from build123d import *

# Parameters (mm, degrees)
SKETCH_1_W      = 35.56
SKETCH_1_H      = 44.45
SKETCH_1_R      = 1.397
EXTRUDE_1_DEPTH = 1.5
SKETCH_2_R      = 7.5
EXTRUDE_2_DEPTH = 15


with BuildPart() as part:
    # 草图1 → 凸台-拉伸1 (new body)
    with BuildSketch(Plane.XY):
        with Locations((0, 22.225)):
            Rectangle(SKETCH_1_W, SKETCH_1_H)
        with Locations((-14.732, 41.45)):
            Circle(SKETCH_1_R, mode=Mode.SUBTRACT)
        with Locations(Location((14.732, 41.45, 0), (0, 0, 180))):
            Circle(SKETCH_1_R, mode=Mode.SUBTRACT)
    extrude(amount=EXTRUDE_1_DEPTH)

    # 草图2 → 凸台-拉伸2 (add)
    with BuildSketch(Plane.XY.offset(1.5)):
        with Locations((0, 35)):
            Circle(SKETCH_2_R)
    extrude(amount=EXTRUDE_2_DEPTH)


solid = part.part
Can you work these out from the model? Positions are in its coordinate system, mm. Coordinates: 2 decimals unless noted, no trailing zeros. Order: outer loops, then holes, each group sorted by start corner. A loop starts at its lowest first (then second) coordinate and runs counter-clockwise, first axis right, second up. Notation, with made-up numbers: (-1, 76) - (47, 76) arc R23 cw to (47, 99) - close; hole circle Ø9 at (86.25, 26). An arc over 180 degrees is marked (long way). Answer as a JSON object with one key per item and string values. Group by question number.
Q1. I need wall thicknesses on line 1 (Z direction, x = 15.5, y = 31.5); line 2 (Y direction, x = -6, z = 10.25); line 3 (X direction, y = 32, z = 10). Which ranges of each line are inside material? Lowest first, please. Write a range as from..to.
Q2. Imagine slicing it at C-C (y = 35). Please give me the cut outline in (x, z).
Q3. We'd pull the mould along Y, two halves only. Please class faces 1 (the face through (-1.63, 27.68, 8.9)), 2 (the face through (17.78, 22, 1)), 3 (the face through (14.914, 40.065, 0.74)), 4 (the face through (-16.128, 41.511, 0.74)): +Y half, -Y half, draft (parallel to the pull), parting line (faces both ways), or undercut.
Q4. Will these pins go through, and if not, where does the flat tip stop? P1, Ø2, axis at x = -5.5, y = 24.5, coming from the +Z side; P2, Ø8, axis at x = 9.5, z = 8.5, coming from the -Y side; P3, Ø1.5, axis at x = 7.5, z = 14.5, coming from the +Y side.
Q5. Imagine slicing it at B-B (x = 0). Please give me the cut outline in (y, z), and give its area (3 significant figures).
Q6. Imagine slicing it at D-D (z = 9). Please give me the cut outline in (x, y), and give its area (3 significant figures).
Q7. Imagine slicing it at A-A (x = 15.5). Please give me the cut outline in (y, z), and give its area (3 significant figures).
Determined:
{
 "1": {"line 1": "z = 0..1.5", "line 2": "y = 30.5..39.5", "line 3": "x = -6.87..6.87"},
 "2": {"outline": "(-17.78, 0) - (17.78, 0) - (17.78, 1.5) - (7.5, 1.5) - (7.5, 16.5) - (-7.5, 16.5) - (-7.5, 1.5) - (-17.78, 1.5) - close"},
 "3": {"face 1": "parting line", "face 2": "draft", "face 3": "undercut", "face 4": "undercut"},
 "4": {"P1": "stops at z = 1.5", "P2": "stops at y = 29.9", "P3": "stops at y = 38.27"},
 "5": {"outline": "(0, 0) - (44.45, 0) - (44.45, 1.5) - (42.5, 1.5) - (42.5, 16.5) - (27.5, 16.5) - (27.5, 1.5) - (0, 1.5) - close", "area": "292 mm2"},
 "6": {"outline": "circle Ø15 at (0, 35)", "area": "177 mm2"},
 "7": {"outline": "(0, 0) - (40.28, 0) - (40.28, 1.5) - (0, 1.5) - close; (42.62, 0) - (44.45, 0) - (44.45, 1.5) - (42.62, 1.5) - close", "area": "63.2 mm2"}
}
